Here's how the part is built. I have some questions about the finished solid (model axes, mm). A direction names the side the tool comes from. Give positions to 0.01 mm unless a question says otherwise; leave off trailing zeros. Order: outer loops, then holes, each group sorted by start corner. A loop starts at its lowest first (then second) coordinate and runs counter-clockwise, first axis right, second up. Notation, with made-up numbers: (-7, 76.25) -> (39, 76.25) arc R3 ccw to (39, 80.25) -> close; hole circle Ø1 at (36.5, 48.25). An arc over 180 degrees is marked (long way). Write each question's results on one line, items separated by ' | '. Start each with the question number.
Q1. Thinking about a two-plate mould opening in Y: for faces 4 (the face through (0.28, -0.11, -8.32)), 5 (the face through (0, -6.25, -2)), 6 (the face through (-3.364, 3.004, 12.535)), which applies, pulls with the +Y half, pulls with the -Y half, needs draft (parallel to the pull), parting line crosses it, or undercut?
Q2. For faces 1 (the face through (0, 6.25, -2)), 2 (the face through (20, 1.48, -2.25)), 3 (the face through (-20, 1.48, -2.25)), which set-ups out of +Z, -Z, +X, -X, +Y, -Y let a thin tool reach every point of the face, with its end or its side?
Q3. Imagine slicing it at B-B, the plane y = 0. Please give me the cut outline in (x, z), then the cut area to 3 significant figures.
Q4. Imagine slicing it at A-A, the plane x = 0.5. Please give me the cut outline in (y, z), then the cut area to 3 significant figures.
Q5. Imagine slicing it at C-C, the plane z = 2. Please give me the cut outline in (x, y).
Q6. I need wall thicknesses on line 1 along Z through (x, y) = (29.5, 2.5); line 2 along Z through (x, y) = (22, 1.75); line 3 along Y through (x, z) = (-13.5, -3). Which ranges of each line are inside material? Lowest first, please. Write a range as [from, to].
Q7. I'm going to push flat-ended pins straight in: pin 1 (1.5 mm diameter, centred on x = 23, z = 43, fed in from -Y); pin 2 (4 mm diameter, centred on x = -10.5, y = 9, fed in from -Z); pin 3 (12 mm diameter, centred on y = -9.5, z = 22.5, fed in from -X); pin 4 (5 mm diameter, centred on x = 7.5, y = 1.5, fed in from -Z). Where does each tip first touch, or does it pass through?
Q8. Imagine slicing it at D-D, the plane x = 22.5. Please give me the cut outline in (y, z), then the cut area to 3 significant figures.
```python
from build123d import *

# Parameters (mm, degrees)
BOSS_EXTRUDE1_DEPTH = 5
BOSS_EXTRUDE2_DEPTH = 5
BOSS_EXTRUDE3_DEPTH = 5
SKETCH5_R           = 10
SKETCH5_R_2         = 7.5
CUT_EXTRUDE1_DEPTH  = 5
SKETCH6_R           = 10.366071997
BOSS_EXTRUDE4_DEPTH = 35
SKETCH7_R           = 7.5
CUT_EXTRUDE2_DEPTH  = 5
BOSS_EXTRUDE5_DEPTH = 40
SKETCH10_R          = 2.25
CUT_EXTRUDE3_DEPTH  = 40


with BuildPart() as part:
    # Sketch1 → Boss-Extrude1 (new body)
    with BuildSketch(Plane.XY):
        with BuildLine():
            Line((-20, 12.5), (20, 12.5))
            ThreePointArc((20, 12.5), (32.5, 0), (20, -12.5))
            Line((20, -12.5), (-20, -12.5))
            ThreePointArc((-20, -12.5), (-32.5, 0), (-20, 12.5))
        make_face()
    extrude(amount=BOSS_EXTRUDE1_DEPTH)

    # Sketch2 → Boss-Extrude2 (add)
    with BuildSketch(Plane.XY.offset(5)):
        with BuildLine():
            Line((-20, 12.5), (20, 12.5))
            ThreePointArc((20, 12.5), (32.5, 0), (20, -12.5))
            Line((20, -12.5), (-20, -12.5))
            ThreePointArc((-20, -12.5), (-32.5, 0), (-20, 12.5))
        make_face()
    extrude(amount=BOSS_EXTRUDE2_DEPTH)

    # Sketch4 → Boss-Extrude3 (add)
    with BuildSketch(Plane.XY.offset(10)):
        with BuildLine():
            Line((-20, 12.5), (20, 12.5))
            ThreePointArc((20, 12.5), (32.5, 0), (20, -12.5))
            Line((20, -12.5), (-20, -12.5))
            ThreePointArc((-20, -12.5), (-32.5, 0), (-20, 12.5))
        make_face()
    extrude(amount=BOSS_EXTRUDE3_DEPTH)

    # Sketch5 → Cut-Extrude1 (cut)
    with BuildSketch(Plane.XY.offset(15)):
        with Locations((-12.902032685, 0)):
            Circle(SKETCH5_R)
        with Locations((-12.902032685, 0)):
            Circle(SKETCH5_R_2, mode=Mode.SUBTRACT)
    extrude(amount=-CUT_EXTRUDE1_DEPTH, mode=Mode.SUBTRACT)

    # Sketch6 → Boss-Extrude4 (add)
    with BuildSketch(Plane.XY.offset(15)):
        with Locations((14.874986592, 0)):
            Circle(SKETCH6_R)
    extrude(amount=BOSS_EXTRUDE4_DEPTH)

    # Sketch7 → Cut-Extrude2 (cut)
    with BuildSketch(Plane.XY.offset(15)):
        with Locations((-12.902032685, 0)):
            Circle(SKETCH7_R)
    extrude(amount=-CUT_EXTRUDE2_DEPTH, mode=Mode.SUBTRACT)

    # Sketch9 → Boss-Extrude5 (add)
    with BuildSketch(Plane(origin=(20, 0, 0), x_dir=(0, 0, -1), z_dir=(1, 0, 0))):
        with BuildLine():
            Line((0, 6.25), (0, 0))
            Line((0, 0), (0, -6.25))
            Line((0, -6.25), (4.5, -6.25))
            ThreePointArc((4.5, -6.25), (8.319298262, 0), (4.5, 6.25))
            Line((4.5, 6.25), (0, 6.25))
        make_face()
    extrude(amount=-BOSS_EXTRUDE5_DEPTH)

    # Sketch10 → Cut-Extrude3 (cut)
    with BuildSketch(Plane(origin=(20, 0, 0), x_dir=(0, 0, -1), z_dir=(1, 0, 0))):
        with Locations((4.159649131, 0)):
            Circle(SKETCH10_R)
    extrude(amount=-CUT_EXTRUDE3_DEPTH, mode=Mode.SUBTRACT)


solid = part.part
```
Geometry check:
1) face 4: parting line crosses it | face 5: pulls with the -Y half | face 6: undercut
2) face 1: -Z, +X, -X, +Y | face 2: -Z, +X, +Y, -Y | face 3: -Z, -X, +Y, -Y
3) outline: (-32.5, 0) -> (-20, 0) -> (-20, -1.91) -> (20, -1.91) -> (20, 0) -> (32.5, 0) -> (32.5, 15) -> (25.24, 15) -> (25.24, 50) -> (4.51, 50) -> (4.51, 15) -> (-2.9, 15) -> (-2.9, 10) -> (-22.9, 10) -> (-22.9, 15) -> (-32.5, 15) -> close; (-20, -8.32) -> (20, -8.32) -> (20, -6.41) -> (-20, -6.41) -> close | area: 1,750 mm²
4) outline: (-12.5, 0) -> (-6.25, 0) -> (-6.25, -4.5) arc R7.02 ccw to (6.25, -4.5) -> (6.25, 0) -> (12.5, 0) -> (12.5, 15) -> (-12.5, 15) -> close; hole circle Ø4.5 at (0, -4.16) | area: 449 mm²
5) outline: (-20, -12.5) -> (20, -12.5) arc R12.5 ccw to (20, 12.5) -> (-20, 12.5) arc R12.5 ccw to start
6) line 1: [0, 15] | line 2: [0, 50] | line 3: [-6.25, -1.93], [1.93, 6.25]
7) pin 1: y = -7.28 | pin 2: z = 0 | pin 3: x = 5.12 | pin 4: z = -8.32
8) outline: (-12.25, 0) -> (12.25, 0) -> (12.25, 15) -> (7.02, 15) -> (7.02, 50) -> (-7.02, 50) -> (-7.02, 15) -> (-12.25, 15) -> close | area: 859 mm²
